Work out the finished part from the listing and answer in its coordinate system (mm). A direction names the side the tool comes from. Round coordinates to 2 decimals unless told otherwise and drop trailing zeros. Loops run counter-clockwise (first coordinate to the right, second up) from the corner with the lowest first, then second, coordinate; pieces in that order, holes last.
```python
from build123d import *

# Parameters (mm, degrees)
SKETCH_1_W          = 55
SKETCH_1_H          = 39
EXTRUDE_1_DEPTH     = 2
SKETCH_2_W          = 23
SKETCH_2_H          = 6
EXTRUDE_2_DEPTH     = 2
SKETCH_3_W          = 6
SKETCH_3_H          = 5
EXTRUDE_3_DEPTH     = 11
SKETCH_5_R          = 0.95
CUT_EXTRUDE_1_DEPTH = 11
SKETCH_6_W          = 55
SKETCH_6_H          = 0.541458129
EXTRUDE_4_DEPTH     = 8
SKETCH_8_R          = 1.65
EXTRUDE_6_DEPTH     = 2
SKETCH_10_W         = 3
SKETCH_10_H         = 6
EXTRUDE_7_DEPTH     = 8
SKETCH_11_R         = 1.5
CUT_EXTRUDE_3_DEPTH = 13
SKETCH_12_R         = 3
EXTRUDE_8_DEPTH     = 7.5
SKETCH_13_W         = 10
SKETCH_13_H         = 3.7
EXTRUDE_9_DEPTH     = 1
FILLET_3_RADIUS     = 3
FILLET_3_LENGTH     = 3
SKETCH_15_R         = 1.75
CUT_EXTRUDE_5_DEPTH = 23
SKETCH_16_W         = 15.5
SKETCH_16_H         = 4
EXTRUDE_10_DEPTH    = 20
SKETCH_17_R         = 1.5
EXTRUDE_11_DEPTH    = 10
FILLET_4_R          = 10
SKETCH_18_W         = 26.564734734
SKETCH_18_H         = 10.454508508
CUT_EXTRUDE_6_DEPTH = 10
CUT_EXTRUDE_7_DEPTH = 8
CUT_EXTRUDE_8_DEPTH = 8
FILLET_6_R          = 5
SKETCH_21_R         = 1.4
CUT_EXTRUDE_9_DEPTH = 4
FILLET_7_R          = 10


with BuildPart() as part:
    # 草图1 → 凸台-拉伸1 (new body)
    with BuildSketch(Plane(origin=(0, 0, 0), x_dir=(1, 0, 0), z_dir=(0, 1, 0))):
        Rectangle(SKETCH_1_W, SKETCH_1_H)
    extrude(amount=EXTRUDE_1_DEPTH)

    # 草图2 → 凸台-拉伸2 (add)
    with BuildSketch(Plane(origin=(0, 2, 0), x_dir=(1, 0, 0), z_dir=(0, 1, 0))):
        with Locations((0, -22.5)):
            Rectangle(SKETCH_2_W, SKETCH_2_H)
    extrude(amount=-EXTRUDE_2_DEPTH)

    # 草图3 → 凸台-拉伸3 (add)
    with BuildSketch(Plane(origin=(0, 2, 0), x_dir=(1, 0, 0), z_dir=(0, 1, 0))):
        with Locations((-9, -12.341458129)):
            Rectangle(SKETCH_3_W, SKETCH_3_H)
        with Locations((-9, 16.458541871)):
            Rectangle(SKETCH_3_W, SKETCH_3_H)
    extrude(amount=EXTRUDE_3_DEPTH)

    # 草图5 → 切除-拉伸1 (cut)
    with BuildSketch(Plane.ZY.offset(12)):
        with Locations((-15.908541871, 9.5)):
            Circle(SKETCH_5_R)
        with Locations((11.791458129, 9.5)):
            Circle(SKETCH_5_R)
    extrude(amount=-CUT_EXTRUDE_1_DEPTH, mode=Mode.SUBTRACT)

    # 草图6 → 凸台-拉伸4 (add)
    with BuildSketch(Plane(origin=(0, 2, 0), x_dir=(1, 0, 0), z_dir=(0, 1, 0))):
        with Locations((0, 19.229270936)):
            Rectangle(SKETCH_6_W, SKETCH_6_H)
    extrude(amount=EXTRUDE_4_DEPTH)

    # 草图8 → 凸台-拉伸6 (add, symmetric)
    with BuildSketch(Plane(origin=(0, 0, 0), x_dir=(0, 0, -1), z_dir=(1, 0, 0))):
        with BuildLine():
            Line((28.189872998, 17), (28.189872998, 0))
            Line((28.189872998, 0), (18.189872998, 0))
            Line((18.189872998, 0), (18.189872998, 17))
            ThreePointArc((18.189872998, 17), (23.189872998, 22), (28.189872998, 17))
        make_face()
        with Locations((23.189872998, 17)):
            Circle(SKETCH_8_R, mode=Mode.SUBTRACT)
    extrude(amount=EXTRUDE_6_DEPTH, both=True)

    # 草图10 → 凸台-拉伸7 (add)
    with BuildSketch(Plane(origin=(0, 2, 0), x_dir=(1, 0, 0), z_dir=(0, 1, 0))):
        with Locations((0.45, -20.5)):
            Rectangle(SKETCH_10_W, SKETCH_10_H)
    extrude(amount=EXTRUDE_7_DEPTH)

    # 草图11 → 切除-拉伸3 (cut)
    with BuildSketch(Plane.XY.offset(-18.958541871)):
        with Locations((-10, 3)):
            Circle(SKETCH_11_R)
    cut_extrude_3 = extrude(amount=-CUT_EXTRUDE_3_DEPTH, mode=Mode.SUBTRACT)

    # 草图12 → 凸台-拉伸8 (add)
    with BuildSketch(Plane.ZY.offset(27.5)):
        with BuildLine():
            Line((-39.5, -22), (-39.5, 10))
            Line((-39.5, 10), (-19.5, 10))
            Line((-19.5, 10), (-19.5, 0))
            Line((-19.5, 0), (-24.5, 0))
            Line((-24.5, 0), (-24.5, -22))
            ThreePointArc((-24.5, -22), (-32, -29.5), (-39.5, -22))
        make_face()
        with Locations((-32, -22)):
            Circle(SKETCH_12_R, mode=Mode.SUBTRACT)
    extrude_8 = extrude(amount=-EXTRUDE_8_DEPTH)

    # 草图13 → 凸台-拉伸9 (add)
    with BuildSketch(Plane.XZ):
        with Locations((0, 19.15)):
            Rectangle(SKETCH_13_W, SKETCH_13_H)
    extrude(amount=EXTRUDE_9_DEPTH)

    # 镜向1: 切除-拉伸3, 凸台-拉伸8 across plane
    add(cut_extrude_3.mirror(Plane(origin=(0, 0, 0), x_dir=(0, 0, 1), z_dir=(1, 0, 0))), mode=Mode.SUBTRACT)
    add(extrude_8.mirror(Plane(origin=(0, 0, 0), x_dir=(0, 0, 1), z_dir=(1, 0, 0))))

    # 圆角3: full round fillet: the end face becomes a half cylinder, R = half its width
    fillet_3_face = Plane((0.45, 10, 20.5), x_dir=(1, 0, 0), z_dir=(0, 1, 0))  # on the end face: x along it, z out of the body
    fillet_3_slab = fillet_3_face.offset(-FILLET_3_RADIUS / 2) * Box(FILLET_3_LENGTH, 2 * FILLET_3_RADIUS, FILLET_3_RADIUS, mode=Mode.PRIVATE)  # the body's end, R deep
    fillet_3_round = Plane((0.45, 7, 20.5), x_dir=(0, 1, 0), z_dir=(1, 0, 0)) * Cylinder(FILLET_3_RADIUS, FILLET_3_LENGTH, mode=Mode.PRIVATE)  # its axis R under the face
    add(fillet_3_slab - fillet_3_round, mode=Mode.SUBTRACT)

    # 草图15 → 切除-拉伸5 (cut)
    with BuildSketch(Plane.ZY.offset(1.05)):
        with Locations((20.5, 7)):
            Circle(SKETCH_15_R)
    extrude(amount=-CUT_EXTRUDE_5_DEPTH, mode=Mode.SUBTRACT)

    # 草图16 → 凸台-拉伸10 (add)
    with BuildSketch(Plane(origin=(0, 0, -19.5), x_dir=(-1, 0, 0), z_dir=(0, 0, -1))):
        with Locations((0, 8)):
            Rectangle(SKETCH_16_W, SKETCH_16_H)
    extrude(amount=EXTRUDE_10_DEPTH)

    # 草图17 → 凸台-拉伸11 (add)
    # profile 1 of 2: a face of its own
    with BuildSketch(Plane(origin=(0, 0, -19.5), x_dir=(-1, 0, 0), z_dir=(0, 0, -1))):
        Polygon((-20, 0), (-2, 0), (-2, 6), (-7.75, 6), (-7.75, 10), (-20, 10), align=None)
        with Locations(Location((-10, 3, 0), (0, 0, 221.810314896))):
            Circle(SKETCH_17_R, mode=Mode.SUBTRACT)
    # profile 2 of 2: a face of its own
    with BuildSketch(Plane(origin=(0, 0, -19.5), x_dir=(-1, 0, 0), z_dir=(0, 0, -1))):
        Polygon((7.75, 6), (2, 6), (2, 0), (20, 0), (20, 10), (7.75, 10), align=None)
        with Locations(Location((10, 3, 0), (0, 0, 180))):
            Circle(SKETCH_17_R, mode=Mode.SUBTRACT)
    extrude(amount=EXTRUDE_11_DEPTH)

    # 圆角4
    fillet_4_edges = [part.edges().sort_by_distance(p)[0] for p in [
        (23.75, 10, -39.5),
        (-23.75, 10, -39.5),
    ]]
    fillet(fillet_4_edges, radius=FILLET_4_R)

    # 草图18 → 切除-拉伸6 (cut)
    with BuildSketch(Plane(origin=(0, 10, 0), x_dir=(1, 0, 0), z_dir=(0, 1, 0))):
        with Locations((-0.840887807, 36.727254254)):
            Rectangle(SKETCH_18_W, SKETCH_18_H)
    extrude(amount=-CUT_EXTRUDE_6_DEPTH, mode=Mode.SUBTRACT)

    # 草图19 → 切除-拉伸7 (cut)
    with BuildSketch(Plane(origin=(27.5, 0, 0), x_dir=(0, 0, -1), z_dir=(1, 0, 0))):
        Polygon((24.3, 10), (39.5, -19.395601839), (39.5, 10), align=None)
    extrude(amount=-CUT_EXTRUDE_7_DEPTH, mode=Mode.SUBTRACT)

    # 草图20 → 切除-拉伸8 (cut)
    with BuildSketch(Plane.ZY.offset(27.5)):
        Polygon((-24.3, 10), (-39.5, 10), (-39.5, -19.395601839), align=None)
    extrude(amount=-CUT_EXTRUDE_8_DEPTH, mode=Mode.SUBTRACT)

    # 圆角6
    fillet_6_edges = [part.edges().sort_by_distance(p)[0] for p in [
        (-23.75, 0, -24.5),
        (23.75, 0, -24.5),
        (23.5, 10, -24.3),
        (-23.5, 10, -24.3),
    ]]
    fillet(fillet_6_edges, radius=FILLET_6_R)

    # 草图21 → 切除-拉伸9 (cut)
    with BuildSketch(Plane.XZ.offset(1)):
        with Locations(Location((0, 19.15, 0), (0, 0, 270))):
            Circle(SKETCH_21_R)
    extrude(amount=-CUT_EXTRUDE_9_DEPTH, mode=Mode.SUBTRACT)

    # 圆角7
    fillet_7_edges = [part.edges().sort_by_distance(p)[0] for p in [
        (27.5, 1, 19.5),
        (-27.5, 1, 19.5),
    ]]
    fillet(fillet_7_edges, radius=FILLET_7_R)


solid = part.part
```
1. Find section C-C (x = 3). Write down the section's boundary in (y, z).
Answer key:
outline: (-1, 17.3) - (0, 17.3) - (0, -29.5) - (6, -29.5) - (6, -31.5) - (10, -31.5) - (10, -18.96) - (2, -18.96) - (2, 25.5) - (0, 25.5) - (0, 21) - (-1, 21) - close
2. Consider probe 1 along X at (y, z) = (-25, -28.5); probe 2 along Z at (x, y) = (-10, 9); probe 3 along X at (y, z) = (7.5, -18). Determine where each line is inside the solid, lowest interval first.
Answer key:
probe 1: x = -27.5 to -20, 20 to 27.5
probe 2: z = -29.5 to -16.72, -15.1 to -13.96, 9.84 to 10.98, 12.6 to 14.84
probe 3: x = -12 to -6
3. Find section B-B (y = -6). Write down the section's boundary in (x, z).
Answer key:
outline: (-27.5, -32.57) - (-20, -32.57) - (-20, -24.5) - (-27.5, -24.5) - close; (20, -32.57) - (27.5, -32.57) - (27.5, -24.5) - (20, -24.5) - close
4. Determine the mould class of faces 1 (the face through (23.8, -29.5, -31.84)), 2 (the face through (-9, 11, -18.959)), 3 (the face through (14, 1, 19.5)), 4 (the face through (-9, 7, -13.959)) for opening direction Z: +Z half, -Z half, draft (parallel to the pull), parting line (faces both ways), or undercut.
Answer key:
face 1: parting line
face 2: -Z half
face 3: +Z half
face 4: undercut
5. Which of the six approach directions +Z, -Z, +X, -X, +Y, -Y give full straight-line access (tool end or side, diameter ignored) to faces 5 (the face through (1.39, 0.97, 19.33)), 6 (the face through (-6, 7, 12)), 7 (the face through (-4, 6, -18.959)), 8 (the face through (0, 3, -28.19))?
Answer key:
face 5: -Y
face 6: +Z, +X, +Y
face 7: +Z, +Y
face 8: -Z, -Y
6. Given pin 1 (8 mm diameter, centred on x = 3, y = 12, fed in from +Z); pin 2 (3 mm diameter, centred on y = 4, z = 12.5, fed in from +X); pin 3 (12 mm diameter, centred on x = 11, z = 2.5, fed in from +Y), each flat-ended and moving along its own axis, determine where each tip first touches the part or whether it passes through.
Answer key:
pin 1: stops at z = 23.27
pin 2: stops at x = -6
pin 3: stops at y = 2
7. Find section D-D (x = -21.5). Write down the section's boundary in (y, z), then the cut area to 3 significant figures.
Answer key:
outline: (-22, -39.5) - (-19.4, -39.5) - (7.3, -25.7) arc R5 ccw to (10, -21.26) - (10, -18.96) - (2, -18.96) - (2, 18.67) - (0, 18.67) - (0, -19.5) arc R5 cw to (-5, -24.5) - (-22, -24.5) arc R7.5 ccw to start; hole circle Ø6 at (-22, -32)
area: 451 mm2
8. Find section A-A (x = -10). Write down the section's boundary in (y, z), then the cut area to 3 significant figures.
Answer key:
outline: (0, -29.5) - (1.5, -29.5) - (1.5, -18.96) - (4.5, -18.96) - (4.5, -29.5) - (10, -29.5) - (10, -18.96) - (13, -18.96) - (13, -13.96) - (2, -13.96) - (2, 9.84) - (13, 9.84) - (13, 14.84) - (2, 14.84) - (2, 25.5) - (0, 25.5) - close; hole circle Ø1.9 at (9.5, -15.91); hole circle Ø1.9 at (9.5, 11.79)
area: 267 mm2
